```python
from build123d import *

# Parameters (mm, degrees)
SKETCH_W        = 78
SKETCH_H        = 68
PAD_DEPTH       = 4
SKETCH001_W     = 74.4
SKETCH001_H     = 64.4
PAD001_DEPTH    = 2.9
SKETCH002_R     = 4
PAD002_DEPTH    = 11
SKETCH003_R     = 2
POCKET_DEPTH    = 17.901
SKETCH004_R     = 2.75
POCKET001_DEPTH = 6.901
FILLET_R        = 1


with BuildPart() as part:
    # Sketch → Pad (new body)
    with BuildSketch(Plane.XY):
        with Locations((39, 34)):
            Rectangle(SKETCH_W, SKETCH_H)
    extrude(amount=PAD_DEPTH)

    # Sketch001 (on Face6 of Pad) → Pad001 (join)
    with BuildSketch(Plane.XY.offset(4)):
        with Locations((39, 34)):
            Rectangle(SKETCH001_W, SKETCH001_H)
    extrude(amount=PAD001_DEPTH)

    # Sketch002 (on Face11 of Pad001) → Pad002 (join)
    with BuildSketch(Plane.XY.offset(6.9)):
        with Locations((9, 53)):
            Circle(SKETCH002_R)
    extrude(amount=PAD002_DEPTH)

    # Sketch003 (on Face13 of Pad002) → Pocket (cut, through all)
    with BuildSketch(Plane.XY.offset(17.9)):
        with Locations((9, 53)):
            Circle(SKETCH003_R)
    extrude(amount=-POCKET_DEPTH, mode=Mode.SUBTRACT)

    # Sketch004 (on Face13 of Pocket) → Pocket001 (cut, through all)
    with BuildSketch(Plane.XY.offset(6.9)):
        with Locations((53.5, 56.5)):
            Circle(SKETCH004_R)
    extrude(amount=-POCKET001_DEPTH, mode=Mode.SUBTRACT)

    # Fillet
    fillet_edges = [part.edges().sort_by_distance(p)[0] for p in [
        (39, 68, 0),
        (78, 34, 0),
        (78, 68, 2),
        (0, 68, 2),
        (39, 0, 0),
        (0, 34, 0),
        (78, 0, 2),
        (0, 0, 2),
    ]]
    fillet(fillet_edges, radius=FILLET_R)


solid = part.part
```
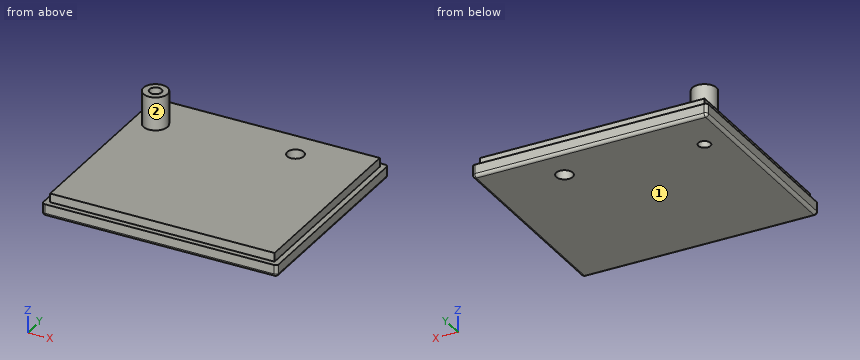
Design review of the part built by this model. Coordinates are the model's own, in mm. Face numbers are marked on the shaded views. A direction names the side the tool comes from. Round coordinates to 2 decimals unless told otherwise and drop trailing zeros. Write each loop counter-clockwise with the first axis right and the second up, starting at its lowest first coordinate (ties: lowest second). Pieces come first, ordered by that corner, then holes.
Item 1: We need section A-A on x = 9. Write out the cut boundary in (y, z).
Item 2: For the marked faces 1 and 2, list the 3-axis set-ups (+Z, -Z, +X, -X, +Y, -Y) from which the entire face can be reached by the end or side of a thin tool; tool diameter is ignored.
Item 3: For probe 1 along Y at (x, z) = (53.5, 4.5); probe 2 along Y at (x, z) = (9, 14); probe 3 along Z at (x, y) = (70, 27.5), list the stretches that pass through material, from the lowest coordinate up.
Item 4: We need section B-B on z = 5.75. Write out the cut boundary in (x, y).
Item 5: Clearance check with flat-ended pins moving along their axes: pin 1 Ø1 at (y, z) = (52.5, 9) entering from +X; pin 2 Ø1.5 at (x, z) = (38.5, 5.5) entering from +Y; pin 3 Ø19.5 at (x, y) = (31.5, 31.5) entering from +Z. State where each tip first meets the part, or that it passes through.
Item 6: We need section C-C on y = 44. Write out the cut boundary in (x, z).
Item 7: We need section D-D on x = 67.5. Write out the cut boundary in (y, z), and give its area (3 significant figures).
Returned:
1. outline: (0, 1) arc R1 ccw to (1, 0) - (51, 0) - (51, 17.9) - (49, 17.9) - (49, 6.9) - (1.8, 6.9) - (1.8, 4) - (0, 4) - close; (55, 0) - (67, 0) arc R1 ccw to (68, 1) - (68, 4) - (66.2, 4) - (66.2, 6.9) - (57, 6.9) - (57, 17.9) - (55, 17.9) - close
2. face 1: -Z, +X, -X, +Y, -Y
2. face 2: +Z
3. probe 1: y = 1.8 to 53.75, 59.25 to 66.2
3. probe 2: y = 49 to 51, 55 to 57
3. probe 3: z = 0 to 6.9
4. outline: (1.8, 1.8) - (76.2, 1.8) - (76.2, 66.2) - (1.8, 66.2) - close; hole circle Ø4 at (9, 53); hole circle Ø5.5 at (53.5, 56.5)
5. pin 1: stops at x = 13
5. pin 2: stops at y = 66.2
5. pin 3: stops at z = 6.9
6. outline: (0, 1) arc R1 ccw to (1, 0) - (77, 0) arc R1 ccw to (78, 1) - (78, 4) - (76.2, 4) - (76.2, 6.9) - (1.8, 6.9) - (1.8, 4) - (0, 4) - close
7. outline: (0, 1) arc R1 ccw to (1, 0) - (67, 0) arc R1 ccw to (68, 1) - (68, 4) - (66.2, 4) - (66.2, 6.9) - (1.8, 6.9) - (1.8, 4) - (0, 4) - close
7. area: 458 mm2
